The figure shows three views and two pictorial views of one solid part (mm, origin at its lowest corner). Answer the questions. Coordinates: 2 decimals unless noted, no trailing zeros. Write each loop counter-clockwise with the first axis right and the second up, starting at its lowest first coordinate (ties: lowest second). Pieces come first, ordered by that corner, then holes. Notation, with made-up numbers: M 1.5,24 L 36.5,24 A27 cw 36.5,50 Z; hole C -25.5,82.25 d10. An arc over 180 degrees is marked long. Write item = value, one per line.
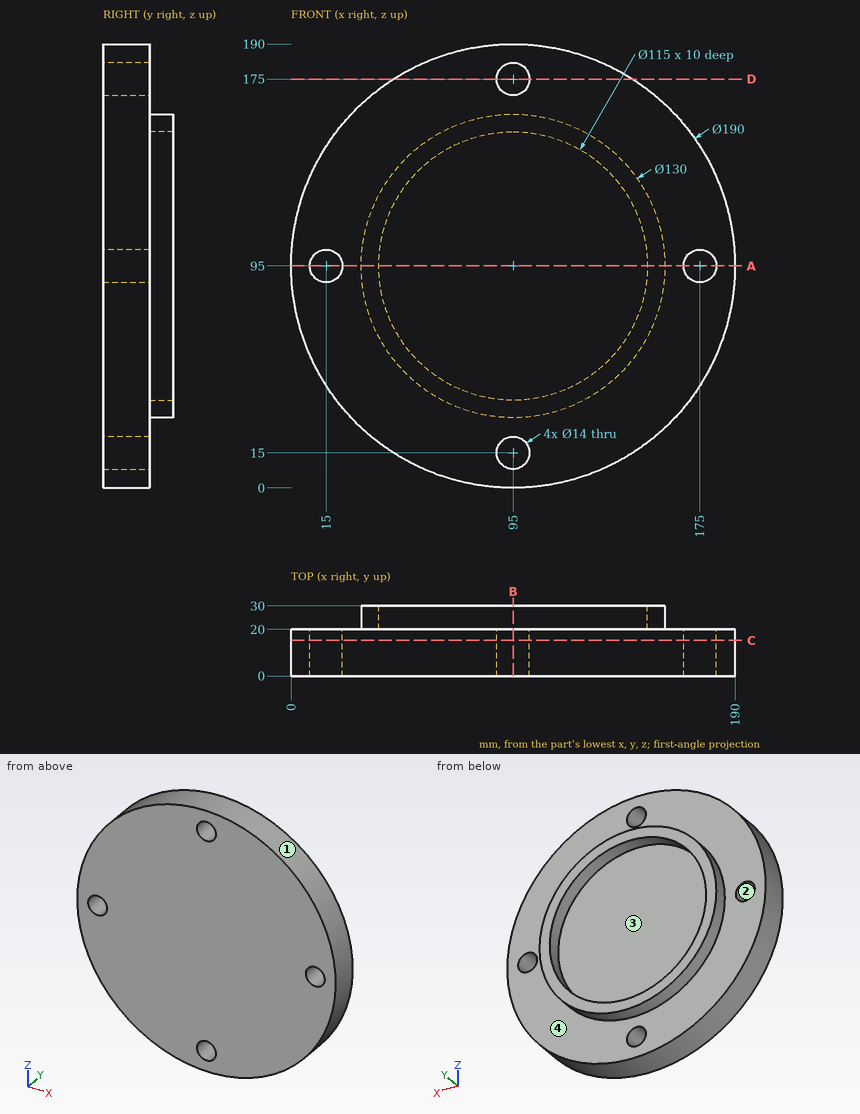
Item 1: Flat-ended cylindrical pins translate along their axes: pin 1 (22.5 mm diameter, centred on x = 95, z = 175, fed in from -Y); pin 2 (12 mm diameter, centred on y = 20.5, z = 144, fed in from +X); pin 3 (3 mm diameter, centred on x = 127.5, y = 19.5, fed in from -Z); pin 4 (8 mm diameter, centred on y = 10.5, z = 143.5, fed in from +X). Find the tip coordinate at first contact, or state that the pin passes through.
Worked answers:
pin_1 = 0
pin_2 = 179.7
pin_3 = 5.2
pin_4 = 178.93
Item 2: Find section B-B (x = 95). Determine the outline of the cut face in (y, z).
Worked answers:
outline = M 0,0 L 20,0 L 20,8 L 0,8 Z; M 0,22 L 20,22 L 20,30 L 30,30 L 30,37.5 L 20,37.5 L 20,152.5 L 30,152.5 L 30,160 L 20,160 L 20,168 L 0,168 Z; M 0,182 L 20,182 L 20,190 L 0,190 Z
Item 3: For a pull along X with two mould halves and no side action, classify the marked faces 1, 2, 3 and 4 as released by +X, released by -X, zero draft, split by the parting line, or undercut.
Worked answers:
face_1 = split by the parting line
face_2 = undercut
face_3 = undercut
face_4 = zero draft
Item 4: Consider line 1 along X through (y, z) = (14.25, 95); line 2 along Y through (x, z) = (144, 51.5); line 3 along Z through (x, y) = (107, 26). Determine where each line is inside the solid, lowest interval first. Write a range as from..to.
Worked answers:
line_1 = 0..8, 22..168, 182..190
line_2 = 0..20
line_3 = 31.12..38.77, 151.23..158.88
Item 5: Find section D-D (z = 175). Determine the outline of the cut face in (x, y), and give its area (3 significant figures).
Worked answers:
outline = M 43.77,0 L 88,0 L 88,20 L 43.77,20 Z; M 102,0 L 146.23,0 L 146.23,20 L 102,20 Z
area = 1,770 mm²
Item 6: Find section A-A (z = 95). Determine the outline of the cut face in (x, y).
Worked answers:
outline = M 0,0 L 8,0 L 8,20 L 0,20 Z; M 22,0 L 168,0 L 168,20 L 160,20 L 160,30 L 152.5,30 L 152.5,20 L 37.5,20 L 37.5,30 L 30,30 L 30,20 L 22,20 Z; M 182,0 L 190,0 L 190,20 L 182,20 Z
Item 7: Find section C-C (y = 15.25). Determine the outline of the cut face in (x, z).
Worked answers:
outline = C 95,95 d190; hole C 15,95 d14; hole C 95,15 d14; hole C 95,175 d14; hole C 175,95 d14
